Design review of the part built by this model. Coordinates are the model's own, in mm. Coordinates: 2 decimals unless noted, no trailing zeros. Write each loop counter-clockwise with the first axis right and the second up, starting at its lowest first coordinate (ties: lowest second). Pieces come first, ordered by that corner, then holes. Notation, with made-up numbers: (-38, -31) - (-30, -31) arc R17 ccw to (-30, -5) - close; hole circle Ø11 at (-3, 49). An arc over 180 degrees is marked (long way). Use a Markdown table: item, result.
from build123d import *

# Parameters (mm, degrees)
F0_R     = 1.55
F1_DEPTH = 5
F2_COUNT = 3
F2_ANGLE = 240


with BuildPart() as f1:
    # F0 (on Top) → F1 (new body)
    with BuildSketch(Plane.XY):
        with BuildLine():
            ThreePointArc((-26.440416, -25.727079), (-24.775, -27.392494), (-22.5, -28.002079))
            Line((-22.5, -28.002079), (22.5, -28.002079))
            ThreePointArc((22.5, -28.002079), (24.775, -27.392494), (26.440416, -25.727079))
            Line((26.440416, -25.727079), (30.970464, -17.880805))
            Line((30.970464, -17.880805), (0, 0))
            Line((0, 0), (-30.970464, -17.880805))
            Line((-30.970464, -17.880805), (-26.440416, -25.727079))
        make_face()
        with Locations((-22.5, -23.452079)):
            Circle(F0_R, mode=Mode.SUBTRACT)
        with Locations((22.5, -23.452079)):
            Circle(F0_R, mode=Mode.SUBTRACT)
    extrude(amount=F1_DEPTH)

    # F2: F1 ×3 about axis
    f2_axis = Axis((0, 0, 2.5), (0, 0, 1))


with BuildPart() as f1_1:
    add(f1.part)
    for i in range(1, F2_COUNT):
        add(f1.part.rotate(f2_axis, i * F2_ANGLE / (F2_COUNT - 1)))


solid = f1_1.part
(1) For L1, parallel to X at y = 30.5, z = 2.55; L2, parallel to X at y = 30, z = 2.5; L3, parallel to X at y = 4, z = 4.6, list the stretches that pass through material, from the lowest coordinate up. Write a range as from..to.
Determined:
| item | result |
|---|---|
| L1 | -14.72..-10.44, -7.68..7.68, 10.44..14.72 |
| L2 | -15.01..-10.03, -8.09..8.09, 10.03..15.01 |
| L3 | -30.02..30.02 |
(2) Draft analysis for pull direction Y (two halves, no side actions). For faces 1 (the cylindrical face through (-24.8, -27.38, 2.46)), 2 (the cylindrical face through (36.11, -7.79, 2.46)), 3 (the cylindrical face through (23.93, -24.05, 2.46)), state which applies: +Y half, -Y half, draft (parallel to the pull), parting line (faces both ways), or undercut.
Determined:
| item | result |
|---|---|
| face 1 | -Y half |
| face 2 | parting line |
| face 3 | undercut |
(3) Take a section at B-B on y = -3.5. Write out the cut boundary in (x, z).
Determined:
| item | result |
|---|---|
| outline | (-34.35, 0) - (34.35, 0) - (34.35, 5) - (-34.35, 5) - close |
(4) For pin 1 (2.5 mm diameter, centred on x = -31.56, y = -7.76, fed in from +Z); pin 2 (4 mm diameter, centred on x = 22.5, y = -23.45, fed in from +Z); pin 3 (1 mm diameter, centred on x = 28.5, z = 4.5, fed in from +Y), all flat-tipped, find the tip position at first contact; note any pin that passes through.
Determined:
| item | result |
|---|---|
| pin 1 | through |
| pin 2 | z = 5 |
| pin 3 | y = 7.51 |
(5) Take a section at C-C on x = 20. Write out the cut boundary in (y, z).
Determined:
| item | result |
|---|---|
| outline | (-28, 0) - (21.36, 0) - (21.36, 5) - (-28, 5) - close |
(6) Take a section at A-A on z = 2.95. Write out the cut boundary in (x, y), and give its area (3 significant figures).
Determined:
| item | result |
|---|---|
| outline | (-35.5, -10.03) - (-26.44, -25.73) arc R4.55 ccw to (-22.5, -28) - (22.5, -28) arc R4.55 ccw to (26.44, -25.73) - (35.5, -10.03) arc R4.55 ccw to (35.5, -5.48) - (13, 33.49) arc R4.55 ccw to (9.06, 35.76) - (-9.06, 35.76) arc R4.55 ccw to (-13, 33.49) - (-35.5, -5.48) arc R4.55 ccw to start; hole circle Ø3.1 at (-31.56, -7.76); hole circle Ø3.1 at (-22.5, -23.45); hole circle Ø3.1 at (-9.06, 31.21); hole circle Ø3.1 at (9.06, 31.21); hole circle Ø3.1 at (22.5, -23.45); hole circle Ø3.1 at (31.56, -7.76) |
| area | 3,310 mm2 |
